from build123d import *

# Parameters (mm, degrees)
CONE002_ROLL_ANGLE = -90
CONE001_ROLL_ANGLE = -90
CONE_ROLL_ANGLE    = 90
BOX_W              = 33
BOX_H              = 3
BOX_DEPTH          = 10
BOX001_W           = 33
BOX001_H           = 3
BOX001_DEPTH       = 10
CYLINDER_R         = 2.25
CYLINDER_DEPTH     = 30
PAD001_DEPTH       = 24
PAD_DEPTH          = 22
CHAMFER_SIZE       = 2
CHAMFER001_SIZE    = 4
CHAMFER002_SIZE    = 4
FILLET_R           = 1
FILLET_PITCH_ANGLE = -90


with BuildPart() as cone002:
    # Cone002 → Cone002 (revolve)
    with BuildSketch(Plane.XZ):
        Polygon((0, 0), (3, 0), (1.75, 3), (0, 3), align=None)
    revolve(axis=Axis((0, 0, 0), (0, 0, 1)))


with BuildPart() as cone002_1:
    # Cone002 roll: moved
    add(cone002.part.rotate(Axis((0, 0, 0), (1, 0, 0)), CONE002_ROLL_ANGLE))


with BuildPart() as cone002_2:
    # Cone002 placement: moved
    add(cone002_1.part.moved(Location((24, -21, -5))))


with BuildPart() as cone001:
    # Cone001 → Cone001 (revolve)
    with BuildSketch(Plane.XZ):
        Polygon((0, 0), (3, 0), (1.75, 3), (0, 3), align=None)
    revolve(axis=Axis((0, 0, 0), (0, 0, 1)))


with BuildPart() as cone001_1:
    # Cone001 roll: moved
    add(cone001.part.rotate(Axis((0, 0, 0), (1, 0, 0)), CONE001_ROLL_ANGLE))


with BuildPart() as cone001_2:
    # Cone001 placement: moved
    add(cone001_1.part.moved(Location((8, -21, -5))))


with BuildPart() as cone:
    # Cone → Cone (revolve)
    with BuildSketch(Plane.XZ):
        Polygon((0, 0), (3, 0), (1.75, 3), (0, 3), align=None)
    revolve(axis=Axis((0, 0, 0), (0, 0, 1)))


with BuildPart() as cone_1:
    # Cone roll: moved
    add(cone.part.rotate(Axis((0, 0, 0), (1, 0, 0)), CONE_ROLL_ANGLE))


with BuildPart() as cone_2:
    # Cone placement: moved
    add(cone_1.part.moved(Location((16.5, 1, -5))))


with BuildPart() as box:
    # Box → Box (new body)
    with BuildSketch(Plane(origin=(0, -2, -10), x_dir=(1, 0, 0), z_dir=(0, 0, 1))):
        with Locations((16.5, 1.5)):
            Rectangle(BOX_W, BOX_H)
    extrude(amount=BOX_DEPTH)


with BuildPart() as box001:
    # Box001 → Box001 (new body)
    with BuildSketch(Plane(origin=(0, -21, -10), x_dir=(1, 0, 0), z_dir=(0, 0, 1))):
        with Locations((16.5, 1.5)):
            Rectangle(BOX001_W, BOX001_H)
    extrude(amount=BOX001_DEPTH)


with BuildPart() as obj1:
    # Cylinder → Cylinder (new body)
    with BuildSketch(Plane(origin=(20, -10, 33), x_dir=(1, 0, 0), z_dir=(0, 0, 1))):
        Circle(CYLINDER_R)
    extrude(amount=CYLINDER_DEPTH)


with BuildPart() as obj2:
    # Sketch001 → Pad001 (new body)
    with BuildSketch(Plane(origin=(20, -10, 36), x_dir=(1, 0, 0), z_dir=(0, 0, 1))):
        Polygon((3.680608, -2.125), (3.680608, 2.125), (0, 4.25), (-3.680608, 2.125), (-3.680608, -2.125), (0, -4.25), align=None)
    extrude(amount=PAD001_DEPTH)


with BuildPart() as bed_holder_cnc:
    # Sketch → Pad (new body)
    with BuildSketch(Plane.XZ.offset(-1)):
        Polygon((0, 0), (33, 0), (10, 23), (10, 33), (30, 33), (30, 42), (10, 42), (10, 54), (30, 54), (30, 63), (0, 63), align=None)
    extrude(amount=PAD_DEPTH)

    # Cut: cut obj2
    add(obj2.part, mode=Mode.SUBTRACT)

    # Cut001: cut obj1
    add(obj1.part, mode=Mode.SUBTRACT)

    # Fusion: union Box, Box001
    add(box.part)
    add(box001.part)

    # Cut002: cut Cone
    add(cone_2.part, mode=Mode.SUBTRACT)

    # Cut003: cut Cone001
    add(cone001_2.part, mode=Mode.SUBTRACT)

    # Cut004: cut Cone002
    add(cone002_2.part, mode=Mode.SUBTRACT)

    # Chamfer
    chamfer_edges = [bed_holder_cnc.edges().sort_by_distance(p)[0] for p in [
        (10, -10, 33),
    ]]
    chamfer(chamfer_edges, length=CHAMFER_SIZE)

    # Chamfer001
    chamfer001_edges = [bed_holder_cnc.edges().sort_by_distance(p)[0] for p in [
        (30, -21, 37.5),
        (30, -21, 58.5),
        (30, 1, 37.5),
        (30, 1, 58.5),
    ]]
    chamfer(chamfer001_edges, length=CHAMFER001_SIZE)

    # Chamfer002
    chamfer002_edges = [bed_holder_cnc.edges().sort_by_distance(p)[0] for p in [
        (0, -10, 63),
    ]]
    chamfer(chamfer002_edges, length=CHAMFER002_SIZE)

    # Fillet
    fillet_edges = [bed_holder_cnc.edges().sort_by_distance(p)[0] for p in [
        (15, -21, 63),
        (2, -21, 61),
        (0, -21, 24.5),
        (16.5, -21, -10),
        (33, -21, -5),
        (21.5, -21, 11.5),
        (10, -21, 27),
        (19, -21, 33),
        (11, -21, 32),
        (15, 1, 63),
        (28, -1, 63),
        (30, -10, 63),
        (28, -19, 63),
        (2, 1, 61),
        (0, 1, 24.5),
        (21.5, 1, 11.5),
        (28, -19, 33),
        (10, 1, 27),
        (19, 1, 33),
        (28, -1, 33),
        (30, -10, 33),
        (11, 1, 32),
        (16.5, 1, -10),
        (33, 1, -5),
    ]]
    fillet(fillet_edges, radius=FILLET_R)


with BuildPart() as bed_holder_cnc_1:
    # Fillet pitch: moved
    add(bed_holder_cnc.part.rotate(Axis((0, 0, 0), (0, 1, 0)), FILLET_PITCH_ANGLE))


with BuildPart() as bed_holder_cnc_2:
    # Fillet placement: moved
    add(bed_holder_cnc_1.part)


solid = bed_holder_cnc_2.part
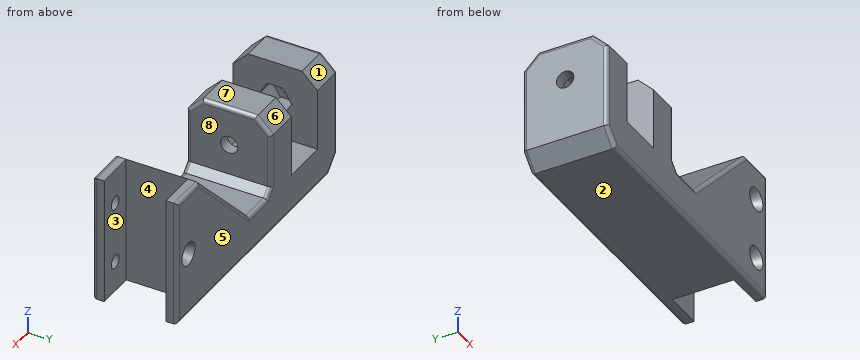
Geometry check sheet. Reference: the model listing, model coordinates, mm. Face numbers are marked on the shaded views. A direction names the side the tool comes from. Round coordinates to 2 decimals unless told otherwise and drop trailing zeros. Loops run counter-clockwise (first coordinate to the right, second up) from the corner with the lowest first, then second, coordinate; pieces in that order, holes last. Notation, with made-up numbers: (-3.75, 28.5) - (49.25, 28.5) arc R25 ccw to (49.25, 64.5) - close; hole circle Ø4 at (-11.5, 79.5). An arc over 180 degrees is marked (long way). One line per question, with ' | ' between items. Start each with the question number.
1. Draft check along Y on the marked faces 1, 2 and 3. Enter one of: released by +Y, released by -Y, zero draft, split by the parting line, or undercut.
2. Cross-section at D-D on x = -48.5. Record the cut outline in (y, z), then the cut area to 3 significant figures.
3. Scan lines: line 1 (Z direction, x = -34.6, y = -10); line 2 (X direction, y = -6, z = 15); line 3 (X direction, y = -13, z = 29.5). Record each from-to range of solid material in increasing order. Write a range as [from, to].
4. Depth check by flat-ended pin: pin 1 (6 mm diameter, centred on x = -49.5, z = 22, fed in from -Y); pin 2 (1.5 mm diameter, centred on x = -54, y = -6.5, fed in from +Z); pin 3 (8 mm diameter, centred on x = -30, y = -18.5, fed in from +Z); pin 4 (3.5 mm diameter, centred on y = -12, z = 18.5, fed in from +X). Enter the tip coordinate at first touch or a pass-through.
5. Cross-section at A-A on z = 8. Record the cut outline in (x, y), then the cut area to 3 significant figures.
6. Cross-section at C-C on x = 5. Record the cut outline in (y, z), then the cut area to 3 significant figures.
7. Tool access check on the marked faces 4, 5, 6, 7 and 8. Record the directions out of +Z, -Z, +X, -X, +Y, -Y that give a thin tool (end or side, any length) a straight path to the whole face; none if there is none.
8. Cross-section at B-B on y = -10. State how many separate pieces and enclosed holes the cut face has, then the cut area to 3 significant figures.
Taken from the geometry:
1) face 1: released by +Y | face 2: zero draft | face 3: undercut
2) outline: (-21, 1) arc R1 ccw to (-20, 0) - (0, 0) arc R1 ccw to (1, 1) - (1, 10) - (-21, 10) - close | area: 220 mm²
3) line 1: [0, 17.75], [22.25, 30] | line 2: [-63, -54], [-42, -33], [-18, 0] | line 3: [-62.87, -54], [-42, -33.13], [-3.5, 0]
4) pin 1: through | pin 2: z = 30 | pin 3: z = 29.95 | pin 4: x = 0
5) outline: (-63, -20) arc R1 ccw to (-62, -21) - (2, -21) - (3.25, -18) - (0, -18) - (0, -2) - (10, -2) - (10, 0) arc R1 ccw to (9, 1) - (-62, 1) arc R1 ccw to (-63, 0) - close; (6.75, -18) - (8, -21) - (9, -21) arc R1 ccw to (10, -20) - (10, -18) - close | area: 1,430 mm²
6) outline: (-21, 1) arc R1 ccw to (-20, 0) - (-18, 0) - (-18, 6.25) - (-21, 5) - close; (-21, 11) - (-18, 9.75) - (-18, 22.25) - (-21, 21) - close; (-21, 27) - (-18, 25.75) - (-18, 33) - (-20, 33) arc R1 ccw to (-21, 32) - close; (-2, 0) - (0, 0) arc R1 ccw to (1, 1) - (1, 13.5) - (-2, 14.75) - close; (-2, 18.25) - (1, 19.5) - (1, 32) arc R1 ccw to (0, 33) - (-2, 33) - close | area: 154 mm²
7) face 4: +Z, -Z, +X | face 5: +Z, -Z, +X, -X, +Y | face 6: +Z, -X, +Y | face 7: +Z, -X, +Y, -Y | face 8: +Z, +Y, -Y
8) separate pieces: 3 | enclosed holes: 0 | area: 1,130 mm²
